Here's how the part is built. I have some questions about the finished solid (model axes, mm). A direction names the side the tool comes from. Give positions to 0.01 mm unless a question says otherwise; leave off trailing zeros. Write each loop counter-clockwise with the first axis right and the second up, starting at its lowest first coordinate (ties: lowest second). Pieces come first, ordered by that corner, then holes. Notation, with made-up numbers: (38.5, 15.5) -> (54.5, 15.5) arc R4 ccw to (54.5, 22.5) -> close; hole circle Ø10 at (69.5, 10.25). An arc over 180 degrees is marked (long way). Use one line per item in the form item = value.
```python
from build123d import *

# Parameters (mm, degrees)
SKETCH_A01_7_R     = 6.85
SKETCH_A01_7_W     = 10
SKETCH_A01_7_H     = 10
EXTRUDE1_DEPTH     = 100
CUT_EXTRUDE1_DEPTH = 101
CUT_EXTRUDE2_DEPTH = 101
CIRPATTERN2_COUNT  = 2
CIRPATTERN2_ANGLE  = 270
SKETCH3_W          = 2
SKETCH3_H          = 1.5
EXTRUDE3_DEPTH     = 100
SKETCH4_W          = 1.5
SKETCH4_H          = 2
EXTRUDE4_DEPTH     = 100


with BuildPart() as part:
    # Sketch A01-7 → Extrude1 (new body)
    with BuildSketch(Plane.XY):
        Polygon((-16.5, -11), (-16.5, -9.5), (-15.863959988, -9.5), (-10.5, -4.136038954), (-10.5, 9.085786), (-12.414214, 11), (-21, 11), (-21, 4), (-25, 4), (-25, 25), (25, 25), (25, -25), (4, -25), (4, -21), (11, -21), (11, -12.414214), (9.085786, -10.5), (-4.136039046, -10.5), (-9.5, -15.863962012), (-9.5, -16.5), (-11, -16.5), (-11, -21), (-4, -21), (-4, -25), (-25, -25), (-25, -4), (-21, -4), (-21, -11), align=None)
        Circle(SKETCH_A01_7_R, mode=Mode.SUBTRACT)
        Polygon((12.414213, -11), (10.500000477, -9.085787477), (10.500000477, 9.085786477), (12.414214, 11), (23, 11), (23, -11), align=None, mode=Mode.SUBTRACT)
        Polygon((11, 12.414213), (9.085787477, 10.500000477), (-9.085786477, 10.500000477), (-11, 12.414214), (-11, 23), (11, 23), align=None, mode=Mode.SUBTRACT)
        with Locations((-18, -18)):
            Rectangle(SKETCH_A01_7_W, SKETCH_A01_7_H, mode=Mode.SUBTRACT)
        with Locations((18, -18)):
            Rectangle(SKETCH_A01_7_W, SKETCH_A01_7_H, mode=Mode.SUBTRACT)
        with Locations((-18, 18)):
            Rectangle(SKETCH_A01_7_W, SKETCH_A01_7_H, mode=Mode.SUBTRACT)
        with Locations((18, 18)):
            Rectangle(SKETCH_A01_7_W, SKETCH_A01_7_H, mode=Mode.SUBTRACT)
    extrude(amount=-EXTRUDE1_DEPTH)

    # Sketch1 → Cut-Extrude1 (cut, through all)
    with BuildSketch(Plane.XY):
        Polygon((-16.5, -13), (-10.707726017, -7.207724875), (-7.207726017, -10.707724185), (-13, -16.49999931), align=None)
    extrude(amount=-CUT_EXTRUDE1_DEPTH, mode=Mode.SUBTRACT)

    # Sketch2 → Cut-Extrude2 (cut, through all)
    with BuildSketch(Plane.XY):
        with BuildLine():
            Line((-9.085786477, 10.500000477), (-6.294899419, 7.650918733))
            ThreePointArc((-6.294899419, 7.650918733), (-0.042574105, 10.257977016), (6.209751208, 7.650918733))
            Line((6.209751208, 7.650918733), (9.085787477, 10.500000477))
            Line((9.085787477, 10.500000477), (-9.085786477, 10.500000477))
        make_face()
    cut_extrude2 = extrude(amount=-CUT_EXTRUDE2_DEPTH, mode=Mode.SUBTRACT)

    # CirPattern2: Cut-Extrude2 ×2 about axis
    cirpattern2_axis = Axis((0, 0, 0), (0, 0, 1))
    for i in range(1, CIRPATTERN2_COUNT):
        add(cut_extrude2.rotate(cirpattern2_axis, i * CIRPATTERN2_ANGLE / (CIRPATTERN2_COUNT - 1)), mode=Mode.SUBTRACT)

    # Sketch3 → Extrude3 (add, through all)
    with BuildSketch(Plane.XY):
        with Locations((-10, 15.75)):
            Rectangle(SKETCH3_W, SKETCH3_H)
        with Locations((10, 15.75)):
            Rectangle(SKETCH3_W, SKETCH3_H)
    extrude(amount=-EXTRUDE3_DEPTH)

    # Sketch4 → Extrude4 (add, through all)
    with BuildSketch(Plane.XY):
        with Locations((15.75, 10)):
            Rectangle(SKETCH4_W, SKETCH4_H)
        with Locations((15.75, -10)):
            Rectangle(SKETCH4_W, SKETCH4_H)
    extrude(amount=-EXTRUDE4_DEPTH)


solid = part.part
```
Q1. I want a section at B-B, the plane x = 5. Write out the boundary of the cut face in (y, z).
Result set:
outline = (-25, -100) -> (-21, -100) -> (-21, 0) -> (-25, 0) -> close; (-10.5, -100) -> (-4.68, -100) -> (-4.68, 0) -> (-10.5, 0) -> close; (4.68, -100) -> (8.67, -100) -> (8.67, 0) -> (4.68, 0) -> close; (23, -100) -> (25, -100) -> (25, 0) -> (23, 0) -> close
Q2. Will these pins go through, and if not, where does the flat tip stop? pin 1 Ø11 at (x, y) = (0, 0) entering from -Z; pin 2 Ø6 at (x, y) = (16, 8.5) entering from -Z.
Result set:
pin_1 = through
pin_2 = -100
Q3. If I drill on line 1 along Y through (x, z) = (0, -41); line 2 along Y through (x, z) = (14, -71), over which ranges is the centre line in solid material (lowest first)? Write a range as from..to.
Result set:
line_1 = -10.5..-6.85, 6.85..10.26, 23..25
line_2 = -25..-23, -13..-11, 11..13, 23..25
Q4. Which directions (+Z, -Z, +X, -X, +Y, -Y) give clear straight access to the entire face, cutting with the end or side of a thin tool? Please do faces 4 (the face through (-25, -15, -49)), 5 (the face through (25, 0, -49)), 6 (the face through (4, -23, -49)), 7 (the face through (18, -13, -49)), 8 (the face through (-23, 4, -49)).
Result set:
face_4 = +Z, -Z, -X, +Y, -Y
face_5 = +Z, -Z, +X, +Y, -Y
face_6 = +Z, -Z, -Y
face_7 = +Z, -Z
face_8 = +Z, -Z, -X
Q5. I want a section at C-C, the plane y = 1. Write out the boundary of the cut face in (x, z), and give its area (3 significant figures).
Result set:
outline = (-10.5, -100) -> (-6.78, -100) -> (-6.78, 0) -> (-10.5, 0) -> close; (6.78, -100) -> (10.21, -100) -> (10.21, 0) -> (6.78, 0) -> close; (23, -100) -> (25, -100) -> (25, 0) -> (23, 0) -> close
area = 915 mm2
Q6. I want a section at A-A, the plane y = 21. Write out the boundary of the cut face in (x, z).
Result set:
outline = (-25, -100) -> (-23, -100) -> (-23, 0) -> (-25, 0) -> close; (-13, -100) -> (-11, -100) -> (-11, 0) -> (-13, 0) -> close; (11, -100) -> (13, -100) -> (13, 0) -> (11, 0) -> close; (23, -100) -> (25, -100) -> (25, 0) -> (23, 0) -> close
Q7. If we mould it in two halves opening along Y, with no side actions, what happens to faces 1 (the face through (-10.1, -13.6, -49.3)), 2 (the face through (-4, -23, -49)), 3 (the face through (0, 25, -49))? For each: +Y half, -Y half, draft (parallel to the pull), parting line (faces both ways), or undercut.
Result set:
face_1 = undercut
face_2 = draft
face_3 = +Y half
Q8. I want a section at D-D, the plane z = -21.5. Count the separate pieces of the cut face and the enclosed holes in it, and give its area (3 significant figures).
Result set:
separate_pieces = 1
enclosed_holes = 7
area = 869 mm2
